Here's how the part is built. I have some questions about the finished solid (model axes, mm). Coordinates: 2 decimals unless noted, no trailing zeros. Loops run counter-clockwise (first coordinate to the right, second up) from the corner with the lowest first, then second, coordinate; pieces in that order, holes last. Notation, with made-up numbers: (57.5, 47) -> (77.5, 47) arc R28 ccw to (77.5, 84) -> close; hole circle Ø10 at (-1, 62). An arc over 180 degrees is marked (long way). Answer as a JSON object with one key per item and string values. Group by question number.
Q1. I want a section at B-B on y = -44.5. Write out the boundary of the cut face in (x, z), then the cut area to 3 significant figures.
Q2. I need wall thicknesses on line 1 (Z direction, x = -11, y = -40); line 2 (Z direction, x = -64.5, y = -4); line 3 (Y direction, x = 48, z = 536). Which ranges of each line are inside material? Lowest first, please.
Q3. I'm going to push flat-ended pins straight in: pin 1 (1.5 mm diameter, centred on x = 57.5, y = 34, fed in from +Z); pin 2 (2 mm diameter, centred on x = 15.5, y = -15, fed in from -Z); pin 3 (6 mm diameter, centred on x = 40, y = -51.5, fed in from -Z). Where does each tip first touch, or does it pass through?
Q4. I want a section at A-A on x = 56. Write out the boundary of the cut face in (y, z).
```python
from build123d import *

# Parameters (mm, degrees)
F0_W     = 150
F0_H     = 150
F1_DEPTH = 587.5
F3_DEPTH = 150


# Not quite as in the source:
# - a pattern or mirror of a feature is missing from the dataset's text; its kind, count and spacing are read off the source's solid


with BuildPart() as f1:
    # F0 (on Top) → F1 (new body, symmetric)
    with BuildSketch(Plane.XY):
        Rectangle(F0_W, F0_H)
    extrude(amount=F1_DEPTH, both=True)

    # F2 (on face) → F3 (cut, through all)
    with BuildSketch(Plane.YZ.offset(75)):
        Polygon((75, 587.5), (-75, 587.5), (75, 500.8974596216), align=None)
    f3 = extrude(amount=-F3_DEPTH, mode=Mode.SUBTRACT)

    # F3_copies: F3 across plane
    add(f3.mirror(Plane(origin=(0, 0, 0), x_dir=(-1, 0, 0), z_dir=(0, 0, -1))), mode=Mode.SUBTRACT)


solid = f1.part
```
Result set:
{
 "1": {"outline": "(-75, -569.89) -> (75, -569.89) -> (75, 569.89) -> (-75, 569.89) -> close", "area": "171,000 mm²"},
 "2": {"line 1": "z = -567.29 to 567.29", "line 2": "z = -546.51 to 546.51", "line 3": "y = -75 to 14.2"},
 "3": {"pin 1": "stops at z = 525", "pin 2": "stops at z = -553.44", "pin 3": "stops at z = -575.66"},
 "4": {"outline": "(-75, -587.5) -> (75, -500.9) -> (75, 500.9) -> (-75, 587.5) -> close"}
}
